Geometry check sheet. Reference: the model listing, model coordinates, mm. Face numbers are marked on the shaded views. Coordinates: 2 decimals unless noted, no trailing zeros. Loops run counter-clockwise (first coordinate to the right, second up) from the corner with the lowest first, then second, coordinate; pieces in that order, holes last.
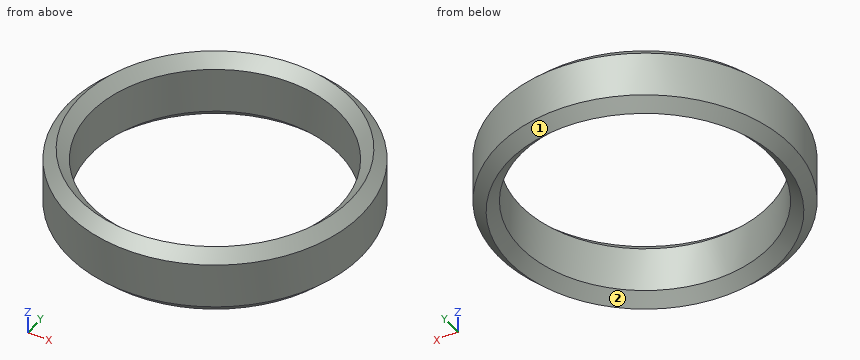
from build123d import *

# Parameters (mm, degrees)
F0_R     = 49.53
F0_R_2   = 41.91
F1_DEPTH = 25.4
F2_SIZE  = 5.08
F4_SIZE  = 5.08


# Not quite as in the source:
# - a fillet or chamfer that OpenCascade refuses, or shapes differently, is made with other operations: its cross-section is extruded or revolved along the edge and cut away or added


with BuildPart() as f1:
    # F0 (on Top) → F1 (new body)
    with BuildSketch(Plane.XY):
        Circle(F0_R)
        Circle(F0_R_2, mode=Mode.SUBTRACT)
    extrude(amount=F1_DEPTH)

    # F2
    f2_edges = [f1.edges().sort_by_distance(p)[0] for p in [
        (-41.91, 0, 25.4),
    ]]
    chamfer(f2_edges, length=F2_SIZE)

    # F3: chamfer of 5.08 on 1 edges, made by hand

    # F3_s1 → F3_t2 (revolve, cut)
    with BuildSketch(Plane.XZ):
        Polygon((44.45, 25.4), (49.53, 20.32), (49.53, 25.4), align=None)
    revolve(axis=Axis((0, 0, 25.4), (0, 0, 1)), mode=Mode.SUBTRACT)

    # F4
    f4_edges = [f1.edges().sort_by_distance(p)[0] for p in [
        (-49.53, 0, 0),
    ]]
    chamfer(f4_edges, length=F4_SIZE)

    # F5: chamfer of 5.08 on 1 edges, made by hand

    # F5_s1 → F5_t2 (revolve, cut)
    with BuildSketch(Plane.XZ):
        Polygon((46.99, 0), (41.91, 5.08), (41.91, 0), align=None)
    revolve(axis=Axis((0, 0, 0), (0, 0, 1)), mode=Mode.SUBTRACT)


solid = f1.part
(1) Sectioned sample at C-C on z = 9.5. Record the cut outline in (x, y), and give its area (3 significant figures).
Findings:
outline: circle Ø99.06 at (0, 0); hole circle Ø83.82 at (0, 0)
area: 2,190 mm2
(2) Scan lines: L1, parallel to Y at x = 0, z = 11.75; L2, parallel to Y at x = -35.5, z = 8; L3, parallel to X at y = -3, z = 11.5. Record each from-to range of solid material in increasing order.
Findings:
L1: y = -49.53 to -41.91, 41.91 to 49.53
L2: y = -34.54 to -22.28, 22.28 to 34.54
L3: x = -49.44 to -41.8, 41.8 to 49.44
(3) Gauge pin test, flat ends, axial feed: pin 1 Ø12 at (x, z) = (-26, 22) entering from +Y; pin 2 Ø1.5 at (x, z) = (-33.5, 14) entering from -Y; pin 3 Ø12 at (y, z) = (-37.5, 13) entering from -X. Record the tip position at first contact, or that the pin passes through.
Findings:
pin 1: stops at y = 45.21
pin 2: stops at y = -37.16
pin 3: stops at x = -38.22
(4) Sectioned sample at A-A on y = 0. Record the cut outline in (x, z).
Findings:
outline: (-49.53, 5.08) - (-45.72, 1.27) - (-41.91, 5.08) - (-41.91, 20.32) - (-45.72, 24.13) - (-49.53, 20.32) - close; (41.91, 5.08) - (45.72, 1.27) - (49.53, 5.08) - (49.53, 20.32) - (45.72, 24.13) - (41.91, 20.32) - close
(5) Draft check along Y on the marked faces 1 and 2. Enter one of: +Y half, -Y half, draft (parallel to the pull), parting line (faces both ways), or undercut.
Findings:
face 1: parting line
face 2: undercut
